Input: part model. Units: mm. Frame: model coordinates. A direction names the side the tool comes from. Round coordinates to 2 decimals unless told otherwise and drop trailing zeros. Loops run counter-clockwise (first coordinate to the right, second up) from the corner with the lowest first, then second, coordinate; pieces in that order, holes last. Notation, with made-up numbers: (58.5, 3) -> (77.5, 3) arc R21 ccw to (77.5, 40) -> close; hole circle Ø2 at (40.5, 41.5). An arc over 180 degrees is marked (long way). Answer as a JSON object with one key per item and string values. Group by question number.
Item 1: Material intervals for line 1 (X direction, y = 18.25, z = -36); line 2 (X direction, y = 25.5, z = -36); line 3 (Y direction, x = -5.25, z = -27), sorted ascending. Write a range as [from, to].
Item 2: Section query C-C on z = -27.5. Return loops of the section in (x, y).
Item 3: Section query D-D on y = 8. Return loops of the section in (x, z).
Item 4: Draft query along Y for faces 4 (the cylindrical face through (-5.36, 21.3, -20.8)), 5 (the flat face through (-14, 29.3, -21)), 6 (the flat face through (-5, 6, -18)), 7 (the cylindrical face through (-12.858, 20.139, -21.395)). Return one class per face: released by +Y, released by -Y, zero draft, split by the parting line, or undercut.
Item 5: Pin query (flat end, axial travel): pin 1 (5 mm diameter, centred on x = -6.5, y = 14.5, fed in from +Z); pin 2 (2 mm diameter, centred on x = -3, y = 16.5, fed in from -Z); pin 3 (10 mm diameter, centred on x = -4.5, z = -19, fed in from +Y). Return the tip coordinate at first contact, or that it passes through.
Item 6: Section query A-A on y = 25.8. Return loops of the section in (x, z).
Item 7: Section query B-B on x = -5.25. Return loops of the section in (y, z).
Item 8: Set-up query: faces 1 (the flat face through (-0.25, 13, -18)), 2 (the flat face through (-5, 13, -16.5)), 3 (the flat face through (3, 29.3, -21)). Return all of +Z, -Z, +X, -X, +Y, -Y with unobstructed straight access to the full face (end or side cutting, diameter ignored); none if empty.
from build123d import *

# Parameters (mm, degrees)
EXTRUDE_1_DEPTH     = 42.2
CUT_EXTRUDE_5_DEPTH = 51.340143027
SKETCH_5_W          = 10
SKETCH_5_H          = 3
EXTRUDE_4_DEPTH     = 14.5
SKETCH_6_W          = 21.5
SKETCH_6_H          = 42.2
EXTRUDE_5_DEPTH     = 7
SKETCH_7_R          = 4.5
CUT_EXTRUDE_3_DEPTH = 42.2
FILLET_2_R          = 2
FILLET_3_R          = 0.5


with BuildPart() as part:
    # 草图2 → 凸台-拉伸1 (new body)
    with BuildSketch(Plane.XY):
        with BuildLine():
            ThreePointArc((2.5, 19.3), (2.207106781, 20.007106781), (1.5, 20.3))
            Line((1.5, 20.3), (-12, 20.3))
            ThreePointArc((-12, 20.3), (-12.707106781, 20.007106781), (-13, 19.3))
            Line((-13, 19.3), (-13, 18.3))
            Line((-13, 18.3), (-12.25, 17.3))
            Line((-12.25, 17.3), (-14.65, 15.5))
            Line((-14.65, 15.5), (-16, 17.3))
            Line((-16, 17.3), (-16, 22.3))
            Line((-16, 22.3), (5.5, 22.3))
            Line((5.5, 22.3), (5.5, 17.3))
            Line((5.5, 17.3), (4.15, 15.5))
            Line((4.15, 15.5), (1.75, 17.3))
            Line((1.75, 17.3), (2.5, 18.3))
            Line((2.5, 18.3), (2.5, 19.3))
        make_face()
    extrude(amount=-EXTRUDE_1_DEPTH)

    # 草图9 → 切除-拉伸5 (cut, through all)
    with BuildSketch(Plane(origin=(0, 0, -42.2), x_dir=(-1, 0, 0), z_dir=(0, 0, -1))):
        with BuildLine():
            Line((-2.7, 18.233333333), (-1.91, 17.18))
            Line((-1.91, 17.18), (-1.75, 17.3))
            Line((-1.75, 17.3), (-2.5, 18.3))
            Line((-2.5, 18.3), (-2.5, 19.3))
            ThreePointArc((-2.5, 19.3), (-2.207106781, 20.007106781), (-1.5, 20.3))
            Line((-1.5, 20.3), (12, 20.3))
            ThreePointArc((12, 20.3), (12.707106781, 20.007106781), (13, 19.3))
            Line((13, 19.3), (13, 18.3))
            Line((13, 18.3), (12.25, 17.3))
            Line((12.25, 17.3), (12.41, 17.18))
            Line((12.41, 17.18), (13.2, 18.233333333))
            Line((13.2, 18.233333333), (13.2, 19.3))
            ThreePointArc((13.2, 19.3), (12.848528137, 20.148528137), (12, 20.5))
            Line((12, 20.5), (-1.5, 20.5))
            ThreePointArc((-1.5, 20.5), (-2.348528137, 20.148528137), (-2.7, 19.3))
            Line((-2.7, 19.3), (-2.7, 18.233333333))
        make_face()
    extrude(amount=-CUT_EXTRUDE_5_DEPTH, mode=Mode.SUBTRACT)

    # 草图5 → 凸台-拉伸4 (add)
    with BuildSketch(Plane.XZ.offset(-20.5)):
        with Locations((-5.25, -18)):
            Rectangle(SKETCH_5_W, SKETCH_5_H)
    extrude(amount=EXTRUDE_4_DEPTH)

    # 草图6 → 凸台-拉伸5 (add)
    with BuildSketch(Plane(origin=(0, 22.3, 0), x_dir=(1, 0, 0), z_dir=(0, 1, 0))):
        with Locations((-5.25, 21.1)):
            Rectangle(SKETCH_6_W, SKETCH_6_H)
    extrude(amount=EXTRUDE_5_DEPTH)

    # 草图7 → 切除-拉伸3 (cut)
    with BuildSketch(Plane.XY):
        with Locations((-5.25, 25.8)):
            Circle(SKETCH_7_R)
    extrude(amount=-CUT_EXTRUDE_3_DEPTH, mode=Mode.SUBTRACT)

    # 圆角2
    fillet_2_edges = [part.edges().sort_by_distance(p)[0] for p in [
        (-2.421572875, 29.3, -21.1),
        (-8.078427125, 29.3, -21.1),
    ]]
    fillet(fillet_2_edges, radius=FILLET_2_R)

    # 圆角3
    fillet_3_edges = [part.edges().sort_by_distance(p)[0] for p in [
        (4.15, 15.5, -21.1),
        (5.5, 17.3, -21.1),
        (-16, 17.3, -21.1),
        (-14.65, 15.5, -21.1),
        (-12.41, 17.18, -21.1),
        (1.91, 17.18, -21.1),
    ]]
    fillet(fillet_3_edges, radius=FILLET_3_R)


solid = part.part
Solved:
{
 "1": {"line 1": "[-16, -13.2], [2.7, 5.5]", "line 2": "[-16, -9.74], [-0.76, 5.5]", "line 3": "[20.5, 21.3]"},
 "2": {"outline": "(-16, 17.47) arc R0.5 ccw to (-15.9, 17.17) -> (-14.95, 15.9) arc R0.5 ccw to (-14.25, 15.8) -> (-12.81, 16.88) arc R0.5 ccw to (-12.71, 17.58) -> (-13.2, 18.23) -> (-13.2, 19.3) arc R1.2 cw to (-12, 20.5) -> (1.5, 20.5) arc R1.2 cw to (2.7, 19.3) -> (2.7, 18.23) -> (2.21, 17.58) arc R0.5 ccw to (2.31, 16.88) -> (3.75, 15.8) arc R0.5 ccw to (4.45, 15.9) -> (5.4, 17.17) arc R0.5 ccw to (5.5, 17.47) -> (5.5, 29.3) -> (1.07, 29.3) arc R2 ccw to (-0.87, 26.84) arc R4.5 cw (long way) to (-9.63, 26.84) arc R2 ccw to (-11.57, 29.3) -> (-16, 29.3) -> close"},
 "3": {"outline": "(-10.25, -19.5) -> (-0.25, -19.5) -> (-0.25, -16.5) -> (-10.25, -16.5) -> close"},
 "4": {"face 4": "undercut", "face 5": "released by +Y", "face 6": "released by -Y", "face 7": "undercut"},
 "5": {"pin 1": "z = -16.5", "pin 2": "z = -19.5", "pin 3": "y = 29.22"},
 "6": {"outline": "(-16, -42.2) -> (-9.75, -42.2) -> (-9.75, 0) -> (-16, 0) -> close; (-0.75, -42.2) -> (5.5, -42.2) -> (5.5, 0) -> (-0.75, 0) -> close"},
 "7": {"outline": "(6, -19.5) -> (20.5, -19.5) -> (20.5, -42.2) -> (21.3, -42.2) -> (21.3, 0) -> (20.5, 0) -> (20.5, -16.5) -> (6, -16.5) -> close"},
 "8": {"face 1": "+Z, -Z, -Y", "face 2": "+Z, -Y", "face 3": "+Z, -Z, +X, -X, +Y"}
}
